from build123d import *
from OCP.BRepFilletAPI import BRepFilletAPI_MakeChamfer

# Parameters (mm, degrees)
SKETCH1_R           = 26
BOSS_EXTRUDE1_DEPTH = 8
SKETCH2_R           = 6.1
CUT_EXTRUDE2_DEPTH  = 3
SKETCH1_11_R        = 3.8
BOSS_EXTRUDE3_DEPTH = 9
FILLET1_R           = 2.5
SKETCH3_R           = 1.15
SKETCH3_R_2         = 1.160199873
CUT_EXTRUDE3_DEPTH  = 6
CHAMFER1_SIZE       = 1
CHAMFER1_SIZE2      = 1.732050808


with BuildPart() as part:
    # Sketch1 → Boss-Extrude1 (new body)
    with BuildSketch(Plane(origin=(0, 0, 0), x_dir=(1, 0, 0), z_dir=(0, 1, 0))):
        with Locations(Location((0, 0, 0), (0, 0, 270))):
            Circle(SKETCH1_R)
    extrude(amount=BOSS_EXTRUDE1_DEPTH)

    # Sketch2 → Cut-Extrude2 (cut)
    with BuildSketch(Plane.XZ):
        with Locations(Location((0, 0, 0), (0, 0, 270))):
            Circle(SKETCH2_R)
    extrude(amount=-CUT_EXTRUDE2_DEPTH, mode=Mode.SUBTRACT)

    # Sketch1_11 → Boss-Extrude3 (add)
    with BuildSketch(Plane(origin=(0, 0, 0), x_dir=(1, 0, 0), z_dir=(0, 1, 0))):
        with Locations(Location((-13.647160877, 13.647160877, 0), (0, 0, 270))):
            Circle(SKETCH1_11_R)
        with Locations(Location((0, 19.3, 0), (0, 0, 270))):
            Circle(SKETCH1_11_R)
        with Locations(Location((13.647160877, 13.647160877, 0), (0, 0, 270))):
            Circle(SKETCH1_11_R)
        with Locations(Location((19.3, 0, 0), (0, 0, 270))):
            Circle(SKETCH1_11_R)
        with Locations(Location((13.647160877, -13.647160877, 0), (0, 0, 270))):
            Circle(SKETCH1_11_R)
        with Locations(Location((0, -19.3, 0), (0, 0, 270))):
            Circle(SKETCH1_11_R)
        with Locations(Location((-13.647160877, -13.647160877, 0), (0, 0, 270))):
            Circle(SKETCH1_11_R)
        with Locations(Location((-19.3, 0, 0), (0, 0, 270))):
            Circle(SKETCH1_11_R)
    extrude(amount=-BOSS_EXTRUDE3_DEPTH)

    # Fillet1
    fillet1_edges = [part.edges().sort_by_distance(p)[0] for p in [
        (0, 0, -26),
        (0, 8, -26),
    ]]
    fillet(fillet1_edges, radius=FILLET1_R)

    # Sketch3 → Cut-Extrude3 (cut)
    with BuildSketch(Plane(origin=(0, 8, 0), x_dir=(1, 0, 0), z_dir=(0, 1, 0))):
        with Locations(Location((-8, 16, 0), (0, 0, 270))):
            Circle(SKETCH3_R)
        with Locations(Location((8, 16, 0), (0, 0, 270))):
            Circle(SKETCH3_R)
        with Locations(Location((-8, 8, 0), (0, 0, 270))):
            Circle(SKETCH3_R)
        with Locations(Location((8, 8, 0), (0, 0, 270))):
            Circle(SKETCH3_R)
        with Locations(Location((-8, -8, 0), (0, 0, 270))):
            Circle(SKETCH3_R)
        with Locations(Location((8, -8, 0), (0, 0, 270))):
            Circle(SKETCH3_R)
        with Locations(Location((-8, -16, 0), (0, 0, 270))):
            Circle(SKETCH3_R)
        with Locations(Location((8, -16, 0), (0, 0, 270))):
            Circle(SKETCH3_R)
        with Locations(Location((-8, 0, 0), (0, 0, 270))):
            Circle(SKETCH3_R)
        with Locations(Location((8, 0, 0), (0, 0, 270))):
            Circle(SKETCH3_R_2)
    extrude(amount=-CUT_EXTRUDE3_DEPTH, mode=Mode.SUBTRACT)

    # Chamfer1: one chamfer whose edges measure the first distance from different faces: ONE call of the kernel's chamfer builder (chamfer() names one face for all edges)
    chamfer1_edges_1 = [part.edges().sort_by_distance(p)[0] for p in [
        (-13.647160877, -9, -17.447160877),
    ]]
    chamfer1_side_1 = [part.faces().sort_by_distance(p)[0] for p in [
        (-13.647160877, -9, -13.647160877),
    ]]
    chamfer1_edges_2 = [part.edges().sort_by_distance(p)[0] for p in [
        (0, -9, -23.1),
    ]]
    chamfer1_side_2 = [part.faces().sort_by_distance(p)[0] for p in [
        (0, -9, -19.3),
    ]]
    chamfer1_edges_3 = [part.edges().sort_by_distance(p)[0] for p in [
        (13.647160877, -9, -17.447160877),
    ]]
    chamfer1_side_3 = [part.faces().sort_by_distance(p)[0] for p in [
        (13.647160877, -9, -13.647160877),
    ]]
    chamfer1_edges_4 = [part.edges().sort_by_distance(p)[0] for p in [
        (19.3, -9, -3.8),
    ]]
    chamfer1_side_4 = [part.faces().sort_by_distance(p)[0] for p in [
        (19.3, -9, 0),
    ]]
    chamfer1_edges_5 = [part.edges().sort_by_distance(p)[0] for p in [
        (13.647160877, -9, 9.847160877),
    ]]
    chamfer1_side_5 = [part.faces().sort_by_distance(p)[0] for p in [
        (13.647160877, -9, 13.647160877),
    ]]
    chamfer1_edges_6 = [part.edges().sort_by_distance(p)[0] for p in [
        (0, -9, 15.5),
    ]]
    chamfer1_side_6 = [part.faces().sort_by_distance(p)[0] for p in [
        (0, -9, 19.3),
    ]]
    chamfer1_edges_7 = [part.edges().sort_by_distance(p)[0] for p in [
        (-13.647160877, -9, 9.847160877),
    ]]
    chamfer1_side_7 = [part.faces().sort_by_distance(p)[0] for p in [
        (-13.647160877, -9, 13.647160877),
    ]]
    chamfer1_edges_8 = [part.edges().sort_by_distance(p)[0] for p in [
        (-19.3, -9, -3.8),
    ]]
    chamfer1_side_8 = [part.faces().sort_by_distance(p)[0] for p in [
        (-19.3, -9, 0),
    ]]
    chamfer1 = BRepFilletAPI_MakeChamfer(part.part.solid().wrapped)
    for e in chamfer1_edges_1:
        chamfer1.Add(CHAMFER1_SIZE, CHAMFER1_SIZE2, e.wrapped, chamfer1_side_1[0].wrapped)  # the first distance lies on this face
    for e in chamfer1_edges_2:
        chamfer1.Add(CHAMFER1_SIZE, CHAMFER1_SIZE2, e.wrapped, chamfer1_side_2[0].wrapped)  # the first distance lies on this face
    for e in chamfer1_edges_3:
        chamfer1.Add(CHAMFER1_SIZE, CHAMFER1_SIZE2, e.wrapped, chamfer1_side_3[0].wrapped)  # the first distance lies on this face
    for e in chamfer1_edges_4:
        chamfer1.Add(CHAMFER1_SIZE, CHAMFER1_SIZE2, e.wrapped, chamfer1_side_4[0].wrapped)  # the first distance lies on this face
    for e in chamfer1_edges_5:
        chamfer1.Add(CHAMFER1_SIZE, CHAMFER1_SIZE2, e.wrapped, chamfer1_side_5[0].wrapped)  # the first distance lies on this face
    for e in chamfer1_edges_6:
        chamfer1.Add(CHAMFER1_SIZE, CHAMFER1_SIZE2, e.wrapped, chamfer1_side_6[0].wrapped)  # the first distance lies on this face
    for e in chamfer1_edges_7:
        chamfer1.Add(CHAMFER1_SIZE, CHAMFER1_SIZE2, e.wrapped, chamfer1_side_7[0].wrapped)  # the first distance lies on this face
    for e in chamfer1_edges_8:
        chamfer1.Add(CHAMFER1_SIZE, CHAMFER1_SIZE2, e.wrapped, chamfer1_side_8[0].wrapped)  # the first distance lies on this face
    add(Compound.cast(chamfer1.Shape()), mode=Mode.REPLACE)


solid = part.part
Read the model definition and answer for the solid it produces. Units are mm, in the model's axes. A direction names the side the tool comes from. Round coordinates to 2 decimals unless told otherwise and drop trailing zeros.
1) For faces 3 (the face through (-12.51, -3.58, -10.02)), 4 (the face through (-8, 2, 0)), 5 (the face through (0, -9, 19)), determine the directions among +Z, -Z, +X, -X, +Y, -Y from which every point of the face is accessible in a straight line to the end or side of a thin tool.
2) Flat-ended cylindrical pins translate along their axes: pin 1 (0.7 mm diameter, centred on x = -8, z = -0.5, fed in from +Y); pin 2 (1.4 mm diameter, centred on x = -8, z = 8, fed in from -Y); pin 3 (10 mm diameter, centred on y = 6, z = 13.5, fed in from +X). Find the tip coordinate at first contact, or state that the pin passes through.
3) The mould has two halves that part along Z. Classify faces 1 (the face through (-19, -9, 0)), 2 (the face through (-5, 0, 5)): released by +Z, released by -Z, zero draft, split by the parting line, or undercut.
4) Straight lines are drawn through the part: L1, parallel to X at y = 4.95, z = 0; L2, parallel to X at y = 3.4, z = -16; L3, parallel to Z at x = -17, y = -3.25. For each, find the intervals that lie inside material, in ascending order.
Resolved:
1. face 3: -Y
1. face 4: +Y
1. face 5: +Z, -Z, +X, -X, -Y
2. pin 1: stops at y = 2
2. pin 2: stops at y = 0
2. pin 3: stops at x = 24.56
3. face 1: zero draft
3. face 2: undercut
4. L1: x = -26 to -9.15, -6.85 to 6.84, 9.16 to 26
4. L2: x = -20.49 to -9.15, -6.85 to 6.85, 9.15 to 20.49
4. L3: z = -15.44 to -11.86, -3.02 to 3.02, 11.86 to 15.44
